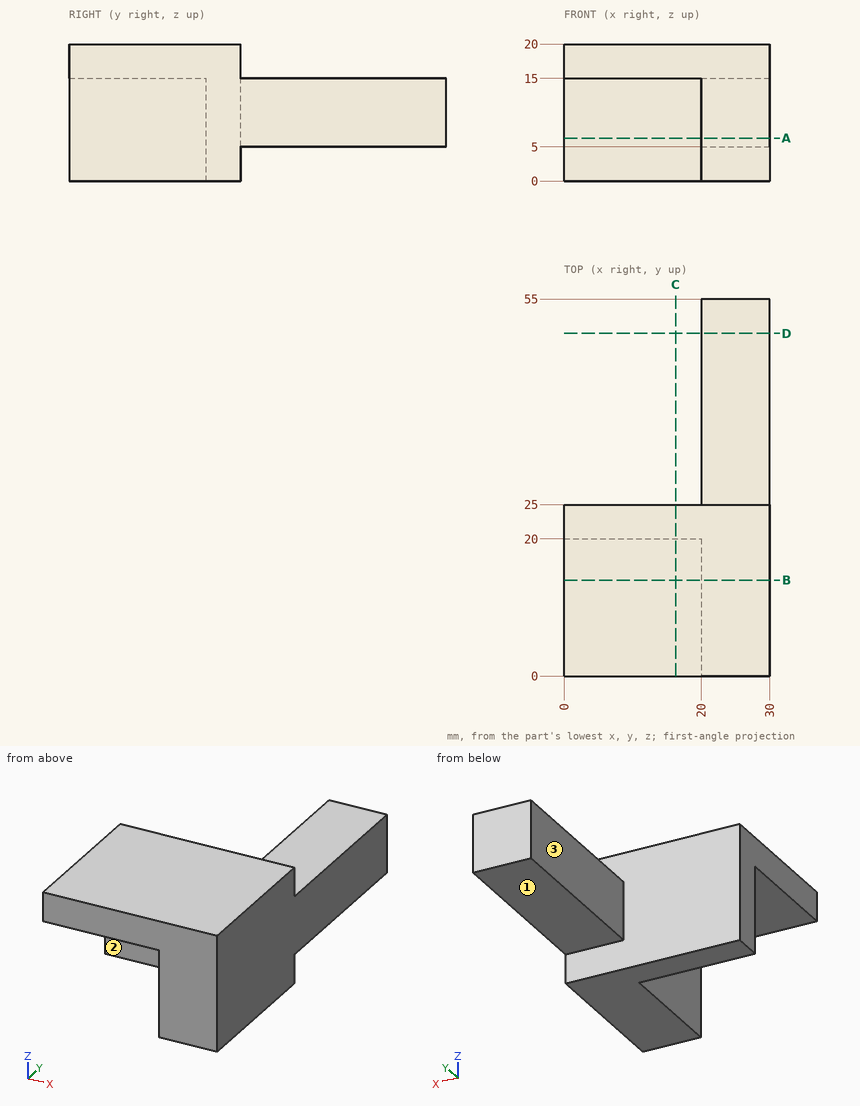
Geometry check sheet. Reference: drawing and pictorial views, mm from the part's lowest x, y, z. A direction names the side the tool comes from. Coordinates: 2 decimals unless noted, no trailing zeros. Order: outer loops, then holes, each group sorted by start corner. A loop starts at its lowest first (then second) coordinate and runs counter-clockwise, first axis right, second up. Notation, with made-up numbers: (-33, 81) - (-3, 81) arc R23 cw to (-3, 119) - close; hole circle Ø5 at (-35, 87.25). An arc over 180 degrees is marked (long way). Answer in a Markdown table with one row per item. Add a question column.
1) Cross-section at C-C, the plane x = 16.25. Record the cut outline in (y, z).
2) Set-up check for the marked faces 1, 2 and 3: record each of +Z, -Z, +X, -X, +Y, -Y from which the full face is reachable in a straight line by a thin tool's end or side.
3) Material ranges on line 1 along X through (y, z) = (16.5, 8.25); line 2 along Z through (x, y) = (21.75, 48); line 3 along Z through (x, y) = (16.75, 14), recorded low to high. Write a range as [from, to].
4) Gauge pin test, flat ends, axial feed: P1, Ø5, axis at x = 22.5, y = 41, coming from the -Z side; P2, Ø11, axis at x = 26, y = 33, coming from the +Z side; P3, Ø10, axis at x = 20.5, z = 17, coming from the -Y side; P4, Ø1.5, axis at x = 9, z = 13.5, coming from the +Y side. Record the tip position at first contact, or that the pin passes through.
5) Cross-section at B-B, the plane y = 14. Record the cut outline in (x, z), then the cut area to 3 significant figures.
6) Cross-section at A-A, the plane z = 6.25. Record the cut outline in (x, y).
7) Cross-section at D-D, the plane y = 50. Record the cut outline in (x, z), then the cut area to 3 significant figures.
Check result:
| question | item | result |
|---|---|---|
| 1 | outline | (0, 15) - (20, 15) - (20, 0) - (25, 0) - (25, 20) - (0, 20) - close |
| 2 | face 1 | -Z, +X, -X, +Y |
| 2 | face 2 | -Z, -X, -Y |
| 2 | face 3 | +Z, -Z, -X, +Y |
| 3 | line 1 | x = [20, 30] |
| 3 | line 2 | z = [5, 15] |
| 3 | line 3 | z = [15, 20] |
| 4 | P1 | stops at z = 5 |
| 4 | P2 | stops at z = 15 |
| 4 | P3 | stops at y = 0 |
| 4 | P4 | stops at y = 25 |
| 5 | outline | (0, 15) - (20, 15) - (20, 0) - (30, 0) - (30, 20) - (0, 20) - close |
| 5 | area | 300 mm² |
| 6 | outline | (0, 20) - (20, 20) - (20, 0) - (30, 0) - (30, 55) - (20, 55) - (20, 25) - (0, 25) - close |
| 7 | outline | (20, 5) - (30, 5) - (30, 15) - (20, 15) - close |
| 7 | area | 100 mm² |
